from build123d import *

# Parameters (mm, degrees)
SKETCH2_R           = 17.55
BOSS_EXTRUDE1_DEPTH = 68.3
SKETCH4_R           = 17.55
SKETCH4_R_2         = 15.85
CUT_EXTRUDE1_DEPTH  = 50
SKETCH5_R           = 2.4
BOSS_EXTRUDE3_DEPTH = 20.1
SKETCH6_W           = 4.602135996
SKETCH6_H           = 1.29181111
CUT_EXTRUDE2_DEPTH  = 12.8
FILLET1_R           = 2


with BuildPart() as part:
    # Sketch2 → Boss-Extrude1 (new body)
    with BuildSketch(Plane.XY):
        Circle(SKETCH2_R)
    extrude(amount=BOSS_EXTRUDE1_DEPTH)

    # Sketch4 → Cut-Extrude1 (cut)
    with BuildSketch(Plane(origin=(0, 0, 0), x_dir=(-1, 0, 0), z_dir=(0, 0, -1))):
        Circle(SKETCH4_R)
        Circle(SKETCH4_R_2, mode=Mode.SUBTRACT)
    extrude(amount=-CUT_EXTRUDE1_DEPTH, mode=Mode.SUBTRACT)

    # Sketch5 → Boss-Extrude3 (add)
    with BuildSketch(Plane.XY.offset(68.3)):
        with Locations((0, -9.25)):
            Circle(SKETCH5_R)
    extrude(amount=BOSS_EXTRUDE3_DEPTH)

    # Sketch6 → Cut-Extrude2 (cut)
    with BuildSketch(Plane.XY.offset(88.4)):
        with Locations((0.017586897, -7.004094445)):
            Rectangle(SKETCH6_W, SKETCH6_H)
    extrude(amount=-CUT_EXTRUDE2_DEPTH, mode=Mode.SUBTRACT)

    # Fillet1
    # the kernel refuses this fillet: 2 mm, written as the material it adds along each edge
    with BuildSketch(Plane(origin=(0, 0, 50), x_dir=(-1, 0, 0), z_dir=(0, -1, 0))) as fillet1_piece_1:
        with BuildLine():
            CenterArc((17.85, 1.977371993), FILLET1_R, 180, 81.373073441)
            Line((15.85, 1.977371993), (15.81, 1.977371993))
            Line((15.81, 1.977371993), (15.81, 0))
            Line((15.81, 0), (15.85, -0.04))
            ThreePointArc((15.85, -0.04), (16.7, -0.04), (17.544, -0.03954744))
            Line((17.544, -0.03954744), (17.55, 0))
        make_face()
    revolve(axis=Axis((0, 0, 50), (0, 0, -1)))


solid = part.part
Source: CAD feature listing. Evaluate the final solid. Frame: model axes, mm. A direction names the side the tool comes from. Round coordinates to 2 decimals unless told otherwise and drop trailing zeros. Loops run counter-clockwise (first coordinate to the right, second up) from the corner with the lowest first, then second, coordinate; pieces in that order, holes last. Notation, with made-up numbers: (-29, -16) -> (12, -16) arc R33 ccw to (12, 14) -> close; hole circle Ø1 at (81.25, -22). An arc over 180 degrees is marked (long way). Answer as a JSON object with one key per item and string values. Group by question number.
Q1. Ray query, line 1 (Z direction, x = -2.5, y = 10.5); line 2 (X direction, y = 0.5, z = 58); line 3 (Y direction, x = -12, z = 32.5). Return the intervals inside material, ascending. Write a range as from..to.
Q2. Section query B-B (y = 0). Output: boundary loops of the cut face in (x, z).
Q3. Section query D-D (z = 71). Output: boundary loops of the cut face in (x, y).
Q4. Section query A-A (x = 0). Output: boundary loops of the cut face in (y, z), plus the area to 3 significant figures.
Q5. Contact query for flat-ended pins moving along their axis: P1, Ø10, axis at x = -10, y = 0.5, coming from the +Z side; P2, Ø12, axis at y = -12, z = 41.5, coming from the -X side; P3, Ø12, axis at x = 13, z = 61, coming from the -Y side. Output: stop coordinate, or through.
Q6. Access query for faces 1 (the cylindrical face through (-0.52, -11.593, 78.209)), 2 (the flat face through (0, -7.65, 82)), 3 (the cylindrical face through (-13.927, -10.679, 59.022)), 4 (the flat face through (0, 0, 0)), 5 (the cylindrical face through (-15.12, 4.76, 23.68)). Directions: +Z, -Z, +X, -X, +Y, -Y. A direction counts if a zero-diameter tool reaches every point of the face in a straight line with its end or side. Return the directions, or none.
Q7. Section query C-C (z = 20.5). Output: boundary loops of the cut face in (x, y).
Completed:
{
 "1": {"line 1": "0..68.3", "line 2": "-17.54..17.54", "line 3": "-10.35..10.35"},
 "2": {"outline": "(-17.55, 50) arc R2 cw to (-15.85, 48.02) -> (-15.85, 0) -> (15.85, 0) -> (15.85, 48.02) arc R2 cw to (17.55, 50) -> (17.55, 68.3) -> (-17.55, 68.3) -> close"},
 "3": {"outline": "circle Ø4.8 at (0, -9.25)"},
 "4": {"outline": "(-17.55, 50) arc R2 cw to (-15.85, 48.02) -> (-15.85, 0) -> (15.85, 0) -> (15.85, 48.02) arc R2 cw to (17.55, 50) -> (17.55, 68.3) -> (-6.85, 68.3) -> (-6.85, 75.6) -> (-7.65, 75.6) -> (-7.65, 88.4) -> (-11.65, 88.4) -> (-11.65, 68.3) -> (-17.55, 68.3) -> close", "area": "2,320 mm²"},
 "5": {"P1": "z = 68.3", "P2": "x = -14.67", "P3": "y = -16.09"},
 "6": {"face 1": "+Z", "face 2": "+Z, +X, -X, +Y", "face 3": "+Z, -Z", "face 4": "-Z, +X, -X, +Y, -Y", "face 5": "-Z"},
 "7": {"outline": "circle Ø31.7 at (0, 0)"}
}
